from build123d import *

# Parameters (mm, degrees)
EXTRUDE_2_DEPTH     = 10
SKETCH_6_R          = 10
CUT_EXTRUDE_2_DEPTH = 10


with BuildPart() as part:
    # Эскиз5 → Бобышка-Вытянуть2 (new body)
    with BuildSketch(Plane.XY):
        Polygon((69.270264014, 2.532805315), (69.270264014, -125.60178411), (-69.270264014, -125.60178411), (-69.270264014, 2.532805315), (-190.995381487, 138.884340659), (190.995381487, 138.884340659), align=None)
        Polygon((-26.270264014, -82.60178411), (26.270264014, -82.60178411), (26.270264014, 18.934099876), (94.96605886, 95.884340659), (-94.96605886, 95.884340659), (-26.270264014, 18.934099876), align=None, mode=Mode.SUBTRACT)
    extrude(amount=EXTRUDE_2_DEPTH)

    # Эскиз6 → Вырез-Вытянуть2 (cut)
    with BuildSketch(Plane.XY.offset(10)):
        with Locations((-146.807623039, 114.578724559)):
            Circle(SKETCH_6_R)
        with Locations((146.807623039, 114.578724559)):
            Circle(SKETCH_6_R)
        with Locations((-50, 0)):
            Circle(SKETCH_6_R)
        with Locations((-50, -100)):
            Circle(SKETCH_6_R)
        with Locations((50, 0)):
            Circle(SKETCH_6_R)
    extrude(amount=-CUT_EXTRUDE_2_DEPTH, mode=Mode.SUBTRACT)


solid = part.part
Read the model definition and answer for the solid it produces. Units are mm, in the model's axes. A direction names the side the tool comes from. Round coordinates to 2 decimals unless told otherwise and drop trailing zeros. Order: outer loops, then holes, each group sorted by start corner. A loop starts at its lowest first (then second) coordinate and runs counter-clockwise, first axis right, second up.
1) The part is cut by section C-C on z = 3.5. Write down the section's boundary in (x, y), plus the area to 3 significant figures.
2) The part is cut by section B-B on y = -100. Write down the section's boundary in (x, z), plus the area to 3 significant figures.
3) The part is cut by section A-A on x = 6.5. Write down the section's boundary in (y, z), plus the area to 3 significant figures.
4) Straight lines are drawn through the part: L1, parallel to X at y = -36.5, z = 3.25; L2, parallel to Y at x = 11, z = 8.5; L3, parallel to Y at x = 50, z = 6.25. For each, find the intervals that lie inside material, in ascending order.
5) The mould has two halves that part along Y. Classify faces 4 (the face through (1, -125.602, 5)), 5 (the face through (69.27, -61, 5)), 6 (the face through (-3, 138.884, 5)), 7 (the face through (136.817, 115.018, 5.07)): released by +Y, released by -Y, zero draft, split by the parting line, or undercut.
6) The part is cut by section D-D on x = -50. Write down the section's boundary in (y, z), plus the area to 3 significant figures.
7) For faces 1 (the face through (60.137, 56.871, 4.93)), 2 (the face through (130.98, 71.66, 4.93)), 3 (the face through (-69.27, -62, 5)), determine the directions among +Z, -Z, +X, -X, +Y, -Y from which every point of the face is accessible in a straight line to the end or side of a thin tool.
8) Flat-ended cylindrical pins translate along their axes: pin 1 (1 mm diameter, centred on y = 108, z = 1, fed in from -X); pin 2 (5 mm diameter, centred on y = -41, z = 4, fed in from +X); pin 3 (5 mm diameter, centred on y = 70.5, z = 7, fed in from -X). Find the tip coordinate at first contact, or state that the pin passes through.
Resolved:
1. outline: (-191, 138.88) - (-69.27, 2.53) - (-69.27, -125.6) - (69.27, -125.6) - (69.27, 2.53) - (191, 138.88) - close; hole circle Ø20 at (-146.81, 114.58); hole (-94.97, 95.88) - (-26.27, 18.93) - (-26.27, -82.6) - (26.27, -82.6) - (26.27, 18.93) - (94.97, 95.88) - close; hole circle Ø20 at (-50, -100); hole circle Ø20 at (-50, 0); hole circle Ø20 at (50, 0); hole circle Ø20 at (146.81, 114.58)
1. area: 37,000 mm2
2. outline: (-69.27, 0) - (-60, 0) - (-60, 10) - (-69.27, 10) - close; (-40, 0) - (69.27, 0) - (69.27, 10) - (-40, 10) - close
2. area: 1,190 mm2
3. outline: (-125.6, 0) - (-82.6, 0) - (-82.6, 10) - (-125.6, 10) - close; (95.88, 0) - (138.88, 0) - (138.88, 10) - (95.88, 10) - close
3. area: 860 mm2
4. L1: x = -69.27 to -26.27, 26.27 to 69.27
4. L2: y = -125.6 to -82.6, 95.88 to 138.88
4. L3: y = -125.6 to -10, 10 to 45.52, 95.88 to 138.88
5. face 4: released by -Y
5. face 5: zero draft
5. face 6: released by +Y
5. face 7: undercut
6. outline: (-125.6, 0) - (-110, 0) - (-110, 10) - (-125.6, 10) - close; (-90, 0) - (-10, 0) - (-10, 10) - (-90, 10) - close; (10, 0) - (45.52, 0) - (45.52, 10) - (10, 10) - close; (95.88, 0) - (138.88, 0) - (138.88, 10) - (95.88, 10) - close
6. area: 1,740 mm2
7. face 1: +Z, -Z
7. face 2: +Z, -Z, +X, -Y
7. face 3: +Z, -Z, -X, -Y
8. pin 1: stops at x = -163.87
8. pin 2: stops at x = 69.27
8. pin 3: stops at x = -132.18
